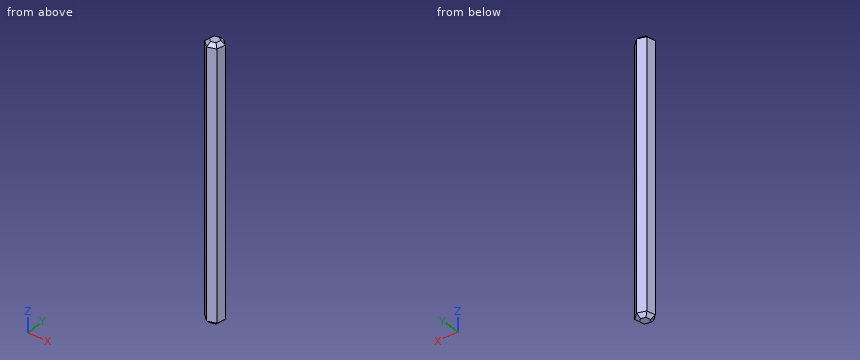
from build123d import *

# Parameters (mm, degrees)
F1_DEPTH = 99.06
F2_SIZE  = 1.27
F3_SIZE  = 1.27


with BuildPart() as f1:
    # F0 (on Top) → F1 (new body)
    with BuildSketch(Plane.XY):
        Polygon((-41.710054, 30.094995), (-38.689673, 31.073729), (-38.027091, 34.178824), (-40.384891, 36.305183), (-43.405272, 35.326448), (-44.067854, 32.221354), align=None)
    extrude(amount=F1_DEPTH)

    # F2
    f2_edges = [f1.edges().sort_by_distance(p)[0] for p in [
        (-40.199863, 30.584362, 0),
        (-38.358382, 32.626277, 0),
        (-39.205991, 35.242004, 0),
        (-41.895082, 35.815816, 0),
        (-43.736563, 33.773901, 0),
        (-42.888954, 31.158174, 0),
    ]]
    chamfer(f2_edges, length=F2_SIZE)

    # F3
    f3_edges = [f1.edges().sort_by_distance(p)[0] for p in [
        (-40.199863, 30.584362, 99.06),
        (-38.358382, 32.626277, 99.06),
        (-39.205991, 35.242004, 99.06),
        (-41.895082, 35.815816, 99.06),
        (-43.736563, 33.773901, 99.06),
        (-42.888954, 31.158174, 99.06),
    ]]
    chamfer(f3_edges, length=F3_SIZE)


solid = f1.part
The listing builds one solid part. Answer for the finished solid, in the listing's coordinates (mm). Round coordinates to 2 decimals unless told otherwise and drop trailing zeros. Order: outer loops, then holes, each group sorted by start corner. A loop starts at its lowest first (then second) coordinate and runs counter-clockwise, first axis right, second up. Notation, with made-up numbers: M 34,65.5 L 49,65.5 A17 ccw 49,97.5 Z; hole C -31,73 d10. An arc over 180 degrees is marked long. Answer in a Markdown table with one row per item. Add a question column.
1) A flat-ended cylindrical pin translates along its axis: pin 1 Ø3 at (y, z) = (35.5, 32) entering from -X. Find the tip coordinate at first contact, or state that the pin passes through.
2) Consider line 1 along Y through (x, z) = (-41, 6); line 2 along Y through (x, z) = (-41.5, 4); line 3 along Z through (x, y) = (-39, 34.75). Determine where each line is inside the solid, lowest interval first. Write a range as from..to.
3) The part is cut by section A-A on z = 10. Determine the outline of the cut face in (x, y) (3 decimals), plus the area to 3 significant figures.
Findings below:
| question | item | result |
|---|---|---|
| 1 | pin 1 | stops at x = -43.69 |
| 2 | line 1 | y = 30.33..36.11 |
| 2 | line 2 | y = 30.16..35.94 |
| 2 | line 3 | z = 1.04..98.02 |
| 3 | outline | M -44.068,32.221 L -41.71,30.095 L -38.69,31.074 L -38.027,34.179 L -40.385,36.305 L -43.405,35.326 Z |
| 3 | area | 26.2 mm² |
